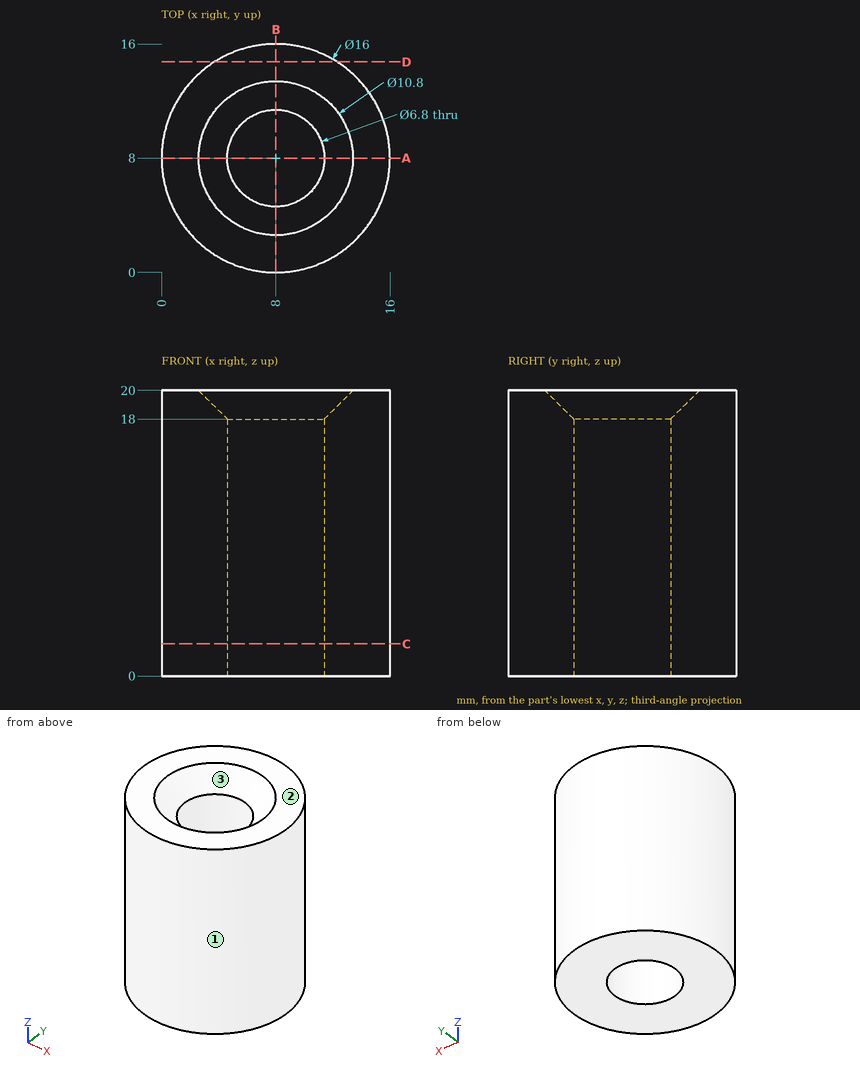
Print and shaded views of the part. All mm, measured from the part's lowest x, y and z. Coordinates: 2 decimals unless noted, no trailing zeros. Loops run counter-clockwise (first coordinate to the right, second up) from the corner with the lowest first, then second, coordinate; pieces in that order, holes last. Notation, with made-up numbers: (-21, 44.5) -> (-9, 44.5) arc R20 ccw to (-9, 53.5) -> close; hole circle Ø4 at (17.5, 79). An arc over 180 degrees is marked (long way). Use one line per item in the form item = value. Start each with the question number.
(1) Cut at C-C on z = 2.25. Give the cut face in (x, y).
(2) Cut at D-D on y = 14.75. Give the cut face in (x, z).
(3) Flat gauge pins, fed straight in: pin 1 (1.5 mm diameter, centred on x = 9, z = 5.5, fed in from -Y); pin 2 (3 mm diameter, centred on x = 10, z = 16.5, fed in from +Y). Where does each tip first touch, or does it go through?
(4) Pull direction Y, two halves, no side cores. Call the marked faces 1, 2 and 3: pulls with the +Y half, pulls with the -Y half, needs draft (parallel to the pull), parting line crosses it, or undercut.
(5) Cut at A-A on y = 8. Give the cut face in (x, z).
(6) Probe probe 1 along Y at (x, z) = (8, 7.25); probe 2 along X at (y, z) = (6.5, 18.25); probe 3 along Y at (x, z) = (4.5, 10). List the from-to ranges inside material, lowest first. Write a range as from..to.
Values:
q1.outline = circle Ø16 at (8, 8); hole circle Ø6.8 at (8, 8)
q2.outline = (3.71, 0) -> (12.29, 0) -> (12.29, 20) -> (3.71, 20) -> close
q3.pin_1 = 0
q3.pin_2 = 15.98
q4.face_1 = parting line crosses it
q4.face_2 = needs draft
q4.face_3 = undercut
q5.outline = (0, 0) -> (4.6, 0) -> (4.6, 18) -> (2.6, 20) -> (0, 20) -> close; (11.4, 0) -> (16, 0) -> (16, 20) -> (13.4, 20) -> (11.4, 18) -> close
q6.probe_1 = 0..4.6, 11.4..16
q6.probe_2 = 0.14..4.67, 11.33..15.86
q6.probe_3 = 0.81..15.19
